Source: CAD feature listing. Evaluate the final solid. Frame: model axes, mm. A direction names the side the tool comes from. Round coordinates to 2 decimals unless told otherwise and drop trailing zeros. Loops run counter-clockwise (first coordinate to the right, second up) from the corner with the lowest first, then second, coordinate; pieces in that order, holes last. Notation, with made-up numbers: (-10.5, 13.25) -> (0.5, 13.25) arc R24 ccw to (0.5, 34.25) -> close; hole circle Ø4 at (58.5, -2). An arc over 180 degrees is marked (long way). Put each result on its own line as item: value. Start each with the question number.
1. Set-up query: faces 1 (the flat face through (-12.038, 4, 4)), 2 (the cylindrical face through (-16.44, -11.21, 0.79)), 3 (the flat face through (12.162, 4, 4)), 4 (the flat face through (11, 5, 5.6)), 5 (the flat face through (0, 17.799, 4)). Return all of +Z, -Z, +X, -X, +Y, -Y with unobstructed straight access to the full face (end or side cutting, diameter ignored); none if empty.
2. Cut plane B-B (y = 3). Return the cut outline in (x, z), then the cut area to 3 significant figures.
3. Draft query along Y for faces 6 (the flat face through (0, 22.949, 1)), 7 (the flat face through (-13, 4, 1.6)), 8 (the flat face through (0, -9.201, 4)). Return one class per face: pulls with the +Y half, pulls with the -Y half, needs draft (parallel to the pull), parting line crosses it, or undercut.
4. Cut plane D-D (z = 0.7). Return the cut outline in (x, y), then the cut area to 3 significant figures.
5. Material intervals for L1, parallel to Y at x = 4, z = 4.3; L2, parallel to X at y = 17, z = 2.9; L3, parallel to Z at x = -5.5, y = 7, sorted ascending.
6. Cut plane C-C (x = 2.5). Return the cut outline in (y, z).
7. Cut plane A-A (z = 2.95). Return the cut outline in (x, y), then the cut area to 3 significant figures.
8. Contact query for flat-ended pins moving along their axis: pin 1 (2 mm diameter, centred on y = 2.5, z = 3, fed in from -X); pin 2 (5 mm diameter, centred on x = 0, y = 13, fed in from +Z); pin 3 (1 mm diameter, centred on x = -12, z = 3, fed in from -Y); pin 4 (2.5 mm diameter, centred on x = 15.25, y = 20.2, fed in from +Z). Output: stop coordinate, or through.
```python
from build123d import *

# Parameters (mm, degrees)
F0_R     = 1.5
F1_DEPTH = 1.6
F2_W     = 24.2
F2_H     = 31
F2_W_2   = 20.2
F2_H_2   = 27
F3_DEPTH = 4


with BuildPart() as f1:
    # F0 (on Top) → F1 (new body)
    with BuildSketch(Plane.XY):
        with BuildLine():
            ThreePointArc((-15.998648, 22.949437), (-17.412861, 22.36365), (-17.998648, 20.949437))
            Line((-17.998648, 20.949437), (-17.998648, -11.050563))
            ThreePointArc((-17.998648, -11.050563), (-17.412861, -12.464777), (-15.998648, -13.050563))
            Line((-15.998648, -13.050563), (16.001352, -13.050563))
            ThreePointArc((16.001352, -13.050563), (17.415566, -12.464777), (18.001352, -11.050563))
            Line((18.001352, -11.050563), (18.001352, 20.949437))
            ThreePointArc((18.001352, 20.949437), (17.415566, 22.36365), (16.001352, 22.949437))
            Line((16.001352, 22.949437), (-15.998648, 22.949437))
        make_face()
        with Locations((-15.248648, -10.300563)):
            Circle(F0_R, mode=Mode.SUBTRACT)
        with Locations((15.251352, -10.300563)):
            Circle(F0_R, mode=Mode.SUBTRACT)
        with Locations((-15.248648, 20.199437)):
            Circle(F0_R, mode=Mode.SUBTRACT)
        with Locations((15.251352, 20.199437)):
            Circle(F0_R, mode=Mode.SUBTRACT)
    extrude(amount=F1_DEPTH)

    # F2 (on face) → F3 (join)
    with BuildSketch(Plane.XY.offset(1.6)):
        with Locations((0.061713, 4.298806)):
            Rectangle(F2_W, F2_H)
        with Locations((0.061713, 4.298806)):
            Rectangle(F2_W_2, F2_H_2, mode=Mode.SUBTRACT)
    extrude(amount=F3_DEPTH)


solid = f1.part
```
Solution:
1. face 1: +Z, -X, +Y, -Y
1. face 2: +Z, -Z
1. face 3: +Z, +X, +Y, -Y
1. face 4: +Z, +X, -X, +Y, -Y
1. face 5: +Z
2. outline: (-18, 0) -> (18, 0) -> (18, 1.6) -> (12.16, 1.6) -> (12.16, 5.6) -> (10.16, 5.6) -> (10.16, 1.6) -> (-10.04, 1.6) -> (-10.04, 5.6) -> (-12.04, 5.6) -> (-12.04, 1.6) -> (-18, 1.6) -> close
2. area: 73.6 mm^2
3. face 6: pulls with the +Y half
3. face 7: needs draft
3. face 8: undercut
4. outline: (-18, -11.05) arc R2 ccw to (-16, -13.05) -> (16, -13.05) arc R2 ccw to (18, -11.05) -> (18, 20.95) arc R2 ccw to (16, 22.95) -> (-16, 22.95) arc R2 ccw to (-18, 20.95) -> close; hole circle Ø3 at (-15.25, -10.3); hole circle Ø3 at (-15.25, 20.2); hole circle Ø3 at (15.25, -10.3); hole circle Ø3 at (15.25, 20.2)
4. area: 1,260 mm^2
5. L1: y = -11.2 to -9.2, 17.8 to 19.8
5. L2: x = -12.04 to -10.04, 10.16 to 12.16
5. L3: z = 0 to 1.6
6. outline: (-13.05, 0) -> (22.95, 0) -> (22.95, 1.6) -> (19.8, 1.6) -> (19.8, 5.6) -> (17.8, 5.6) -> (17.8, 1.6) -> (-9.2, 1.6) -> (-9.2, 5.6) -> (-11.2, 5.6) -> (-11.2, 1.6) -> (-13.05, 1.6) -> close
7. outline: (-12.04, -11.2) -> (12.16, -11.2) -> (12.16, 19.8) -> (-12.04, 19.8) -> close; hole (-10.04, -9.2) -> (10.16, -9.2) -> (10.16, 17.8) -> (-10.04, 17.8) -> close
7. area: 205 mm^2
8. pin 1: stops at x = -12.04
8. pin 2: stops at z = 1.6
8. pin 3: stops at y = -11.2
8. pin 4: passes through
